Check sheet for the modelled part. Datum: model origin and axes. Units: mm. A direction names the side the tool comes from. Round coordinates to 2 decimals unless told otherwise and drop trailing zeros. Loops run counter-clockwise (first coordinate to the right, second up) from the corner with the lowest first, then second, coordinate; pieces in that order, holes last. Notation, with made-up numbers: M -5.75,43 L 34.25,43 A10 ccw 34.25,55 Z; hole C 5,31.25 d8. An arc over 180 degrees is marked long. One line per question, with ' | ' between items. Start each with the question number.
(1) Draft check along X on faces 6 (the face through (-97, -6, 54)), 7 (the face through (38.327, 18.867, 6.961)), 8 (the face through (-38.51, 18.87, 6.28)), 9 (the face through (-91.08, 41.04, 46.95)). Enter one of: +X half, -X half, draft (parallel to the pull), parting line (faces both ways), or undercut.
(2) Thickness scan on probe 1 along Y at (x, z) = (-76, 6.5); probe 2 along X at (y, z) = (41, 53); probe 3 along Y at (x, z) = (-20.5, 6.5). Record the ranges inside material, lowest first. Write a range as [from, to].
(3) Section check B-B (x = -71.5). Record the boundary of the cut face in (y, z).
(4) Section check C-C (z = -11). Record the boundary of the cut face in (x, y).
(5) Section check D-D (x = -97.5). Record the boundary of the cut face in (y, z).
(6) Tool access check on faces 1 (the face through (-111.24, 33.18, 74.84)), 2 (the face through (-91.08, 19.13, 46.95)), 3 (the face through (98, 44, 54)), 4 (the face through (103.92, -2.96, 46.95)), 5 (the face through (103.92, 41.04, 46.95)). Record the directions out of +Z, -Z, +X, -X, +Y, -Y that give a thin tool (end or side, any length) a straight path to the whole face; none if there is none.
(7) Go/stop test with flat-tipped pins: P1, Ø8, axis at x = -12.5, z = 8, coming from the +Y side; P2, Ø1.5, axis at y = 24.5, z = -5.5, coming from the +X side; P3, Ø5, axis at x = 31.5, y = 34.5, coming from the +Z side. Record where each tip stops, or that it passes through.
(8) Section check A-A (y = 22). Record the boundary of the cut face in (x, z), and give its area (3 significant figures).
```python
from build123d import *

# Parameters (mm, degrees)
BOSS_EXTRUDE1_DEPTH = 9.5
BOSS_EXTRUDE2_DEPTH = 19
BOSS_EXTRUDE3_DEPTH = 9.5
SKETCH4_R           = 9.5
CUT_EXTRUDE1_DEPTH  = 151.612195549
BOSS_EXTRUDE4_START = 6
SKETCH4_2_R         = 9.5
BOSS_EXTRUDE4_DEPTH = 50


with BuildPart() as part:
    # Sketch1 → Boss-Extrude1 (new body)
    with BuildSketch(Plane(origin=(0, 0, 0), x_dir=(1, 0, 0), z_dir=(0, 1, 0))):
        with BuildLine():
            ThreePointArc((118.682293684, -40.676118471), (0, 25), (-118.682293684, -40.676118471))
            ThreePointArc((-118.682293684, -40.676118471), (-110.778193938, -75.136606094), (-76.317706316, -67.232506348))
            ThreePointArc((-76.317706316, -67.232506348), (0, -25), (76.317706316, -67.232506348))
            ThreePointArc((76.317706316, -67.232506348), (110.778193938, -75.136606094), (118.682293684, -40.676118471))
        make_face()
    extrude(amount=BOSS_EXTRUDE1_DEPTH)

    # Sketch2 → Boss-Extrude2 (add)
    with BuildSketch(Plane(origin=(0, 9.5, 0), x_dir=(1, 0, 0), z_dir=(0, 1, 0))):
        with BuildLine():
            ThreePointArc((-31.926647669, -30.848128785), (-16.228920494, -26.474094445), (0, -25))
            Line((0, -25), (0, 25))
            ThreePointArc((0, 25), (-22.757218561, 23.138984144), (-44.909728312, 17.605387816))
            Line((-44.909728312, 17.605387816), (-31.926647669, -30.848128785))
        make_face()
        with BuildLine():
            Line((0, 25), (0, -25))
            ThreePointArc((0, -25), (16.228920494, -26.474094445), (31.926647669, -30.848128785))
            Line((31.926647669, -30.848128785), (44.909728312, 17.605387816))
            ThreePointArc((44.909728312, 17.605387816), (22.757218561, 23.138984144), (0, 25))
        make_face()
    extrude(amount=BOSS_EXTRUDE2_DEPTH)

    # Sketch3 → Boss-Extrude3 (add)
    with BuildSketch(Plane(origin=(0, 28.5, 0), x_dir=(1, 0, 0), z_dir=(0, 1, 0))):
        with BuildLine():
            ThreePointArc((-76.317706316, -67.232506348), (-57.097861387, -45.409809383), (-31.926647669, -30.848128785))
            Line((-31.926647669, -30.848128785), (-44.909728312, 17.605387816))
            ThreePointArc((-44.909728312, 17.605387816), (-86.83185423, -5.161009247), (-118.682293684, -40.676118471))
            ThreePointArc((-118.682293684, -40.676118471), (-110.778193938, -75.136606094), (-76.317706316, -67.232506348))
        make_face()
        with BuildLine():
            Line((-44.909728312, 17.605387816), (-31.926647669, -30.848128785))
            ThreePointArc((-31.926647669, -30.848128785), (0, -25), (31.926647669, -30.848128785))
            Line((31.926647669, -30.848128785), (44.909728312, 17.605387816))
            ThreePointArc((44.909728312, 17.605387816), (0, 25), (-44.909728312, 17.605387816))
        make_face()
        with BuildLine():
            Line((44.909728312, 17.605387816), (31.926647669, -30.848128785))
            ThreePointArc((31.926647669, -30.848128785), (57.097861387, -45.409809383), (76.317706316, -67.232506348))
            ThreePointArc((76.317706316, -67.232506348), (110.778193938, -75.136606094), (118.682293684, -40.676118471))
            ThreePointArc((118.682293684, -40.676118471), (86.83185423, -5.161009247), (44.909728312, 17.605387816))
        make_face()
    extrude(amount=BOSS_EXTRUDE3_DEPTH)

    # Sketch4 → Cut-Extrude1 (cut, through all)
    with BuildSketch(Plane(origin=(0, 38, 0), x_dir=(1, 0, 0), z_dir=(0, 1, 0))):
        with Locations(Location((-97.5, -53.95431241, 0), (0, 0, 270))):
            Circle(SKETCH4_R)
        with Locations(Location((97.5, -53.95431241, 0), (0, 0, 270))):
            Circle(SKETCH4_R)
    extrude(amount=-CUT_EXTRUDE1_DEPTH, mode=Mode.SUBTRACT)

    # Sketch4_2 → Boss-Extrude4 (add)
    with BuildSketch(Plane(origin=(0, 38, 0), x_dir=(1, 0, 0), z_dir=(0, 1, 0)).offset(BOSS_EXTRUDE4_START)):
        with Locations(Location((-97.5, -53.95431241, 0), (0, 0, 270))):
            Circle(SKETCH4_2_R)
        with Locations(Location((97.5, -53.95431241, 0), (0, 0, 270))):
            Circle(SKETCH4_2_R)
    extrude(amount=-BOSS_EXTRUDE4_DEPTH)


solid = part.part
```
The answers:
1) face 6: draft | face 7: +X half | face 8: -X half | face 9: undercut
2) probe 1: [0, 9.5], [28.5, 38] | probe 2: [-106.95, -88.05], [88.05, 106.95] | probe 3: [0, 38]
3) outline: M 0,-5.38 L 9.5,-5.38 L 9.5,60.29 L 0,60.29 Z; M 28.5,-5.38 L 38,-5.38 L 38,60.29 L 28.5,60.29 Z
4) outline: M -61.04,0 L 61.04,0 L 61.04,9.5 L 43.14,9.5 L 43.14,28.5 L 61.04,28.5 L 61.04,38 L -61.04,38 L -61.04,28.5 L -43.14,28.5 L -43.14,9.5 L -61.04,9.5 Z
5) outline: M -6,44.45 L 0,44.45 L 0,14.5 L 9.5,14.5 L 9.5,44.45 L 28.5,44.45 L 28.5,14.5 L 38,14.5 L 38,44.45 L 44,44.45 L 44,63.45 L 38,63.45 L 38,78.95 L 28.5,78.95 L 28.5,63.45 L 9.5,63.45 L 9.5,78.95 L 0,78.95 L 0,63.45 L -6,63.45 Z
6) face 1: +Y, -Y | face 2: none | face 3: +Z, -Z, +X, -X, +Y | face 4: -Y | face 5: +Y
7) P1: y = 38 | P2: x = 41.87 | P3: z = 31.66
8) outline: C -97.5,53.95 d19; M -44.91,-17.61 A140.07 ccw 44.91,-17.61 L 31.93,30.85 A90.07 cw -31.93,30.85 Z; C 97.5,53.95 d19 | area: 4,480 mm²
